```python
from build123d import *

# Parameters (mm, degrees)
F1_DEPTH  = 17.5
F3_DEPTH  = 2
F4_R      = 1.3844066796
F4_R_2    = 1.4118495886
F5_DEPTH  = 2
F6_R      = 1.09615194
F6_R_2    = 1.1626457349
F6_R_3    = 1.2756503746
F7_DEPTH  = 4
F9_DEPTH  = 42.8725
F8_W      = 4
F8_H      = 17.0664954185
F8_H_2    = 17.5
F10_DEPTH = 25
F11_R     = 1.09615194
F11_R_2   = 1.1626457349
F11_R_3   = 1.2756503746
F12_DEPTH = 5
F13_W     = 15
F13_H     = 32
F14_DEPTH = 1


with BuildPart() as f1:
    # F0 (on Front) → F1 (new body)
    with BuildSketch(Plane.XZ):
        Polygon((-29.036315158, 133.554469943), (-62.036315158, 133.554469943), (-62.036315158, 118.3553636074), (-79.5507803559, 118.3553636074), (-79.5507803559, 103.6831215024), (-95.036315158, 103.6831215024), (-95.036315158, 69.0787881613), (-79.5507803559, 69.0787881613), (-79.8276141286, 55.2370585501), (-62.036315158, 55.2370585501), (-62.036315158, 43.554469943), (-29.036315158, 43.554469943), (-29.036315158, 66.5872767568), (-34.9804013968, 66.5872767568), (-34.9804013968, 105.6209653616), (-29.036315158, 105.6209653616), align=None)
    extrude(amount=F1_DEPTH)

    # F2 (on face) → F3 (cut)
    with BuildSketch(Plane(origin=(-62.036315158, 0, 0), x_dir=(0, -1, 0), z_dir=(-1, 0, 0))):
        with BuildLine():
            Line((14.58732225, 128.2094269991), (3.0413551722, 128.2094269991))
            ThreePointArc((3.0413551722, 128.2094269991), (1.0878725443, 126.2559443712), (3.0413551722, 124.3024617434))
            Line((3.0413551722, 124.3024617434), (14.58732225, 124.3024617434))
            ThreePointArc((14.58732225, 124.3024617434), (16.5408048779, 126.2559443712), (14.58732225, 128.2094269991))
        make_face()
    extrude(amount=-F3_DEPTH, mode=Mode.SUBTRACT)

    # F4 (on face) → F5 (join)
    with BuildSketch(Plane(origin=(-60.036315158, 0, 0), x_dir=(0, -1, 0), z_dir=(-1, 0, 0))):
        with Locations((5.3467825055, 126.3230890036)):
            Circle(F4_R)
        with Locations((11.7130186409, 126.3377517462)):
            Circle(F4_R_2)
    extrude(amount=F5_DEPTH)

    # F6 (on face) → F7 (cut)
    with BuildSketch(Plane(origin=(-62.036315158, 0, 0), x_dir=(0, -1, 0), z_dir=(-1, 0, 0))):
        with BuildLine():
            Line((13.6235784739, 51.2298978865), (3.7623266689, 51.2298978865))
            ThreePointArc((3.7623266689, 51.2298978865), (2.1155080758, 49.5830792934), (3.7623266689, 47.9362607002))
            Line((3.7623266689, 47.9362607002), (13.6235784739, 47.9362607002))
            ThreePointArc((13.6235784739, 47.9362607002), (15.2703970671, 49.5830792934), (13.6235784739, 51.2298978865))
        make_face()
        with Locations((5.4540927522, 49.5830792934)):
            Circle(F6_R, mode=Mode.SUBTRACT)
        with Locations((8.8431918994, 49.6022440493)):
            Circle(F6_R_2, mode=Mode.SUBTRACT)
        with Locations((12.0892226696, 49.5083071291)):
            Circle(F6_R_3, mode=Mode.SUBTRACT)
    extrude(amount=-F7_DEPTH, mode=Mode.SUBTRACT)

    # F9 (add): a face of the model
    f9_faces = [f1.faces().sort_by_distance(p)[0] for p in [
        (-32.0083582774, -8.75, 105.6209653616),
    ]]
    extrude(f9_faces, amount=F9_DEPTH)

    # F8 (on face) → F10 (cut)
    with BuildSketch(Plane.XZ.offset(17.5)):
        with Locations((-31.036315158, 97.0877176523)):
            Rectangle(F8_W, F8_H)
        with Locations((-31.036315158, 79.804469943)):
            Rectangle(F8_W, F8_H_2)
    extrude(amount=-F10_DEPTH, mode=Mode.SUBTRACT)

    # F11 (on face) → F12 (cut)
    with BuildSketch(Plane(origin=(-80.8999922237, 0, 1.6179950544), x_dir=(0, -1, 0), z_dir=(-0.9998000612, 0, 0.019995942))):
        with BuildLine():
            Line((13.6235784739, 61.979509742), (3.7623266689, 61.979509742))
            ThreePointArc((3.7623266689, 61.979509742), (2.1155080758, 60.3326911488), (3.7623266689, 58.6858725557))
            Line((3.7623266689, 58.6858725557), (13.6235784739, 58.6858725557))
            ThreePointArc((13.6235784739, 58.6858725557), (15.2703970671, 60.3326911488), (13.6235784739, 61.979509742))
        make_face()
        with Locations((5.4540927522, 60.3326911488)):
            Circle(F11_R, mode=Mode.SUBTRACT)
        with Locations((8.8431918994, 60.3326911488)):
            Circle(F11_R_2, mode=Mode.SUBTRACT)
        with Locations((12.0892226696, 60.3326911488)):
            Circle(F11_R_3, mode=Mode.SUBTRACT)
    extrude(amount=-F12_DEPTH, mode=Mode.SUBTRACT)

    # F13 (on face) → F14 (cut)
    with BuildSketch(Plane(origin=(-95.036315158, 0, 0), x_dir=(0, -1, 0), z_dir=(-1, 0, 0))):
        with Locations((8.7, 86.4831215024)):
            Rectangle(F13_W, F13_H)
    extrude(amount=-F14_DEPTH, mode=Mode.SUBTRACT)


solid = f1.part
```
Model file for the job. Use its own axes, mm. A direction names the side the tool comes from. Give positions to 0.01 mm unless a question says otherwise; leave off trailing zeros. Order: outer loops, then holes, each group sorted by start corner. A loop starts at its lowest first (then second) coordinate and runs counter-clockwise, first axis right, second up.
1) Saw through at B-B, the plane x = -85.5. Write the cut outline in (y, z), then the cut area to 3 significant figures.
2) Mould opens along Z. For faces 1 (the cylindrical face through (-61.02, -11.41, 124.96)), 2 (the flat face through (-55, -17.5, 89)), 3 (the flat face through (-46, -9, 43.554)) say: +Z half, -Z half, draft (parallel to the pull), parting line (faces both ways), or undercut.
3) Wall check: probe 1 along Z at (x, y) = (-71, -11.75); probe 2 along X at (y, z) = (-13.75, 111); probe 3 along X at (y, z) = (-14, 86). Give the ranges that are in metal, low to high.
4) Saw through at C-C, the plane z = 109.5. Write the cut outline in (x, y), then the cut area to 3 significant figures.
5) Saw through at A-A, the plane z = 87. Write the cut outline in (x, y).
6) 3-axis set-ups, long thin cutter, end or side, ignore diameter. For faces 4 (the cylindrical face through (-77.24, -7.92, 61.18)), 5 (the flat face through (-62.036, -9, 129)), 6 (the flat face through (-94.036, -9, 87)): which of +Z, -Z, +X, -X, +Y, -Y reach the whole face in a straight line?
7) Pin check, flat tips, straight feed: pin 1 (1.8 mm diameter, centred on y = -5, z = 50, fed in from -X); pin 2 (8 mm diameter, centred on x = -73, y = -15.5, fed in from +Z); pin 3 (10 mm diameter, centred on y = -5, z = 76.5, fed in from +X). Stop position of each tip, or through.
Computed:
1. outline: (-17.5, 69.08) - (0, 69.08) - (0, 103.68) - (-17.5, 103.68) - close
1. area: 606 mm2
2. face 1: undercut
2. face 2: draft
2. face 3: -Z half
3. probe 1: z = 55.24 to 118.36
3. probe 2: x = -79.55 to -29.04
3. probe 3: x = -94.04 to -33.04
4. outline: (-79.55, -17.5) - (-29.04, -17.5) - (-29.04, 0) - (-79.55, 0) - close
4. area: 884 mm2
5. outline: (-95.04, -17.5) - (-33.04, -17.5) - (-33.04, 0) - (-95.04, 0) - (-95.04, -1.2) - (-94.04, -1.2) - (-94.04, -16.2) - (-95.04, -16.2) - close
6. face 4: none
6. face 5: +Z, -X, +Y, -Y
6. face 6: -X
7. pin 1: stops at x = -62.04
7. pin 2: stops at z = 118.36
7. pin 3: stops at x = -33.04
